```python
from build123d import *

# Parameters (mm, degrees)
BOSS_EXTRUDE1_DEPTH      = 20
BOSS_EXTRUDE1_2_DEPTH    = 20
SKETCH2_R                = 73.2
BOSS_EXTRUDE2_DEPTH      = 2
BODY_DELETE_KEEP_1_DEPTH = 22
BOSS_EXTRUDE3_DEPTH      = 1.5
BOSS_EXTRUDE3_DEPTH_BACK = 1.5
FILLET2_R                = 1.5


# Read off the part's stored shape, not the designer's step: Body-Delete/Keep 1
with BuildPart() as part:
    # Sketch1 → Boss-Extrude1 (new body)
    with BuildSketch(Plane(origin=(0, 0, 0), x_dir=(1, 0, 0), z_dir=(0, 1, 0))):
        with BuildLine():
            Line((62.2, -17.8), (-62.2, -17.8))
            Line((-62.2, -17.8), (-62.2, -34.649675323))
            ThreePointArc((-62.2, -34.649675323), (0, -71.2), (62.2, -34.649675323))
            Line((62.2, -34.649675323), (62.2, -17.8))
        make_face()
        with BuildLine():
            Line((60.2, -34.126236241), (60.2, -19.8))
            Line((60.2, -19.8), (-60.2, -19.8))
            Line((-60.2, -19.8), (-60.2, -34.126236241))
            ThreePointArc((-60.2, -34.126236241), (0, -69.2), (60.2, -34.126236241))
        make_face(mode=Mode.SUBTRACT)
    extrude(amount=BOSS_EXTRUDE1_DEPTH)

    # Sketch2 → Boss-Extrude2 (add)
    with BuildSketch(Plane(origin=(0, 20, 0), x_dir=(1, 0, 0), z_dir=(0, 1, 0))):
        with Locations(Location((0, 0, 0), (0, 0, 270))):
            Circle(SKETCH2_R)
    extrude(amount=BOSS_EXTRUDE2_DEPTH)


with BuildPart() as body_2:
    # Sketch1 → Boss-Extrude1 2 (new body)
    with BuildSketch(Plane(origin=(0, 0, 0), x_dir=(1, 0, 0), z_dir=(0, 1, 0))):
        with BuildLine():
            Line((-62.2, -15.8), (62.2, -15.8))
            Line((62.2, -15.8), (62.2, 34.649675323))
            ThreePointArc((62.2, 34.649675323), (0, 71.2), (-62.2, 34.649675323))
            Line((-62.2, 34.649675323), (-62.2, -15.8))
        make_face()
        with BuildLine():
            Line((-60.2, 34.126236241), (-60.2, -13.8))
            Line((-60.2, -13.8), (60.2, -13.8))
            Line((60.2, -13.8), (60.2, 34.126236241))
            ThreePointArc((60.2, 34.126236241), (0, 69.2), (-60.2, 34.126236241))
        make_face(mode=Mode.SUBTRACT)
    extrude(amount=BOSS_EXTRUDE1_2_DEPTH)


with BuildPart() as body_3:
    # Split1: the piece on the far side of the plane
    add(part.part)
    split(bisect_by=Plane(origin=(0, 0, 16.8), x_dir=(-1, 0, 0), z_dir=(0, 0, -1)), keep=Keep.BOTTOM)

    # Sketch4 → Boss-Extrude3 (add, two sides: drawn at the far end of the back side and taken through both)
    with BuildSketch(Plane.XY.offset(39.8).offset(-BOSS_EXTRUDE3_DEPTH_BACK)):
        with BuildLine():
            Line((-9.5, 15.435211288), (-9.5, 27.581262171))
            ThreePointArc((-9.5, 27.581262171), (0, 37.081262171), (9.5, 27.581262171))
            Line((9.5, 27.581262171), (9.5, 15.435211288))
            ThreePointArc((9.5, 15.435211288), (0, 5.935211288), (-9.5, 15.435211288))
        make_face()
        with BuildLine():
            ThreePointArc((-6.5, 15.435211288), (0, 8.935211288), (6.5, 15.435211288))
            Line((6.5, 15.435211288), (6.5, 27.581262171))
            ThreePointArc((6.5, 27.581262171), (0, 34.081262171), (-6.5, 27.581262171))
            Line((-6.5, 27.581262171), (-6.5, 15.435211288))
        make_face(mode=Mode.SUBTRACT)
    extrude(amount=BOSS_EXTRUDE3_DEPTH + BOSS_EXTRUDE3_DEPTH_BACK)

    # Fillet2
    fillet2_edges = [body_3.edges().sort_by_distance(p)[0] for p in [
        (-9.5, 17.717605644, 41.3),
        (0, 5.935211288, 41.3),
        (9.5, 17.717605644, 41.3),
        (-6.5, 17.717605644, 41.3),
        (0, 8.935211288, 41.3),
        (6.5, 17.717605644, 41.3),
        (9.5, 17.717605644, 38.3),
        (6.5, 17.717605644, 38.3),
        (0, 8.935211288, 38.3),
        (-6.5, 17.717605644, 38.3),
        (0, 5.935211288, 38.3),
        (-9.5, 17.717605644, 38.3),
        (9.5, 24.790631086, 38.3),
        (0, 37.081262171, 38.3),
        (-9.5, 24.790631086, 38.3),
        (-9.5, 24.790631086, 41.3),
        (9.5, 24.790631086, 41.3),
        (6.5, 24.790631086, 41.3),
        (-6.5, 24.790631086, 41.3),
        (0, 34.081262171, 41.3),
        (0, 37.081262171, 41.3),
    ]]
    fillet(fillet2_edges, radius=FILLET2_R - 0.0001)  # a hair under: the kernel refuses the full size


with BuildPart() as part_1:
    add(part.part)

    # Split1
    split(bisect_by=Plane(origin=(0, 0, 16.8), x_dir=(-1, 0, 0), z_dir=(0, 0, -1)), keep=Keep.TOP)


with BuildPart() as body_delete_keep_1_tool:
    # Body-Delete/Keep 1 outline → Body-Delete/Keep 1 (new body)
    with BuildSketch(Plane(origin=(0, 0, 0), x_dir=(1, 0, 0), z_dir=(0, 1, 0))):
        with BuildLine():
            ThreePointArc((71.246052522, -16.8), (0, 73.2), (-71.246052522, -16.8))
            Line((-71.246052522, -16.8), (71.246052522, -16.8))
        make_face()
    extrude(amount=BODY_DELETE_KEEP_1_DEPTH)


with BuildPart() as part_2:
    add(part_1.part)

    # Body-Delete/Keep 1: cut by body_delete_keep_1_tool
    add(body_delete_keep_1_tool.part, mode=Mode.SUBTRACT)


with BuildPart() as body_2_1:
    add(body_2.part)

    # Body-Delete/Keep 1: cut by body_delete_keep_1_tool
    add(body_delete_keep_1_tool.part, mode=Mode.SUBTRACT)


solid = body_3.part
```
Here's how the part is built. I have some questions about the finished solid (model axes, mm). A direction names the side the tool comes from. Coordinates: 2 decimals unless noted, no trailing zeros. Order: outer loops, then holes, each group sorted by start corner. A loop starts at its lowest first (then second) coordinate and runs counter-clockwise, first axis right, second up. Notation, with made-up numbers: (9, 28) - (28, 28) arc R32 ccw to (28, 54) - close; hole circle Ø7 at (-40, 60). An arc over 180 degrees is marked (long way). One line per question, with ' | ' between items. Start each with the question number.
1. If we section it at C-C (x = -21): Write out the boundary of the cut face in (y, z).
2. Which directions (+Z, -Z, +X, -X, +Y, -Y) give clear straight access to the entire face, cutting with the end or side of a thin tool? Please do faces 1 (the flat face through (62.2, 10, 26)), 2 (the flat face through (-60.2, 10, 27)), 3 (the flat face through (1, 10, 17.8)), 4 (the flat face through (2, 34, 38.3)).
3. I'm going to push flat-ended pins straight in: pin 1 Ø11 at (x, y) = (2, 26) entering from -Z; pin 2 Ø4.5 at (y, z) = (8.5, 29) entering from -X; pin 3 Ø8 at (y, z) = (13.5, 24.5) entering from +X; pin 4 Ø17 at (x, z) = (-13.5, 53.5) entering from +Y. Where does each tip first touch, or does it pass through?
4. If we section it at D-D (y = 12): Give the number of separate pieces and of enclosed holes in the cut face, and give its area (3 significant figures).
5. If we mould it in two halves opening along Y, with no side actions, what happens to faces 5 (the cylindrical face through (0.14, 34.08, 39.04)), 6 (the flat face through (0, 0, 19)), 7 (the cylindrical face through (-1.059, 9.86, 71.192))? For each: released by +Y, released by -Y, zero draft, split by the parting line, or undercut.
6. Please list where these lines run through material, in increasing order: line 1 along Y through (x, z) = (8, 62); line 2 along X through (y, z) = (12.5, 61); line 3 along Z through (x, y) = (-24, 5). Write a range as [from, to].
7. If we section it at B-B (z = 27): Write out the boundary of the cut face in (x, y).
Model answer:
1) outline: (0, 17.8) - (20, 17.8) - (20, 16.8) - (22, 16.8) - (22, 70.12) - (20, 70.12) - (20, 68.03) - (0, 68.03) - (0, 65.94) - (20, 65.94) - (20, 19.8) - (0, 19.8) - close
2) face 1: +Z, -Z, +X, -Y | face 2: -Y | face 3: -Z, +X, -X, -Y | face 4: -Z, +X, -X, +Y
3) pin 1: stops at z = 16.8 | pin 2: stops at x = -62.2 | pin 3: stops at x = 62.2 | pin 4: stops at y = 22
4) separate pieces: 3 | enclosed holes: 1 | area: 620 mm²
5) face 5: undercut | face 6: released by -Y | face 7: zero draft
6) line 1: y = [20, 22] | line 2: x = [-36.72, -32.67], [32.67, 36.72] | line 3: z = [17.8, 19.8], [64.9, 67.03]
7) outline: (-68.04, 20) - (-62.2, 20) - (-62.2, 0) - (-60.2, 0) - (-60.2, 20) - (60.2, 20) - (60.2, 0) - (62.2, 0) - (62.2, 20) - (68.04, 20) - (68.04, 22) - (-68.04, 22) - close
